Can you work these out from the drawing? Everything is in mm from the part's minimum corner. Round coordinates to 2 decimals unless told otherwise and drop trailing zeros. Order: outer loops, then holes, each group sorted by start corner. A loop starts at its lowest first (then second) coordinate and runs counter-clockwise, first axis right, second up. Notation, with made-up numbers: (74.25, 58.5) -> (115.25, 58.5) arc R28 cw to (115.25, 92.5) -> close; hole circle Ø7 at (-19.5, 80.5). An arc over 180 degrees is marked (long way). One line per item, written item: value.
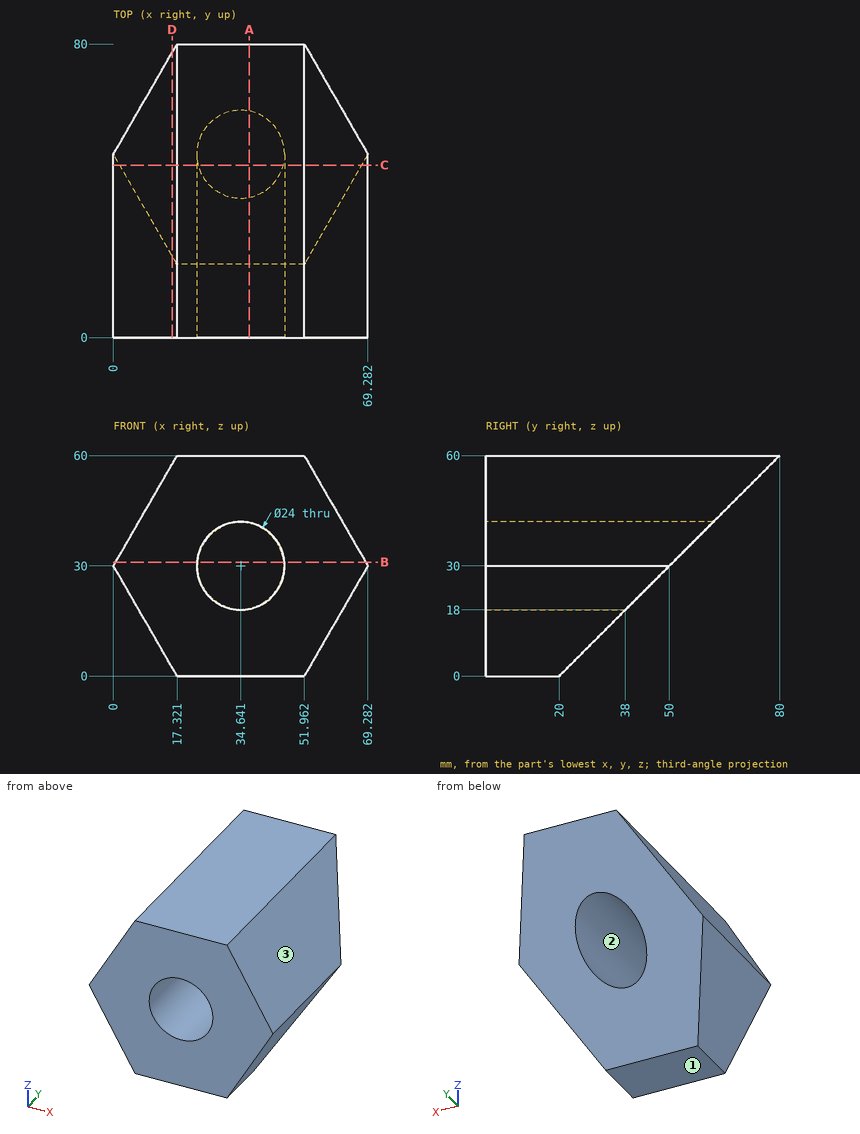
Q1. For P1, Ø4, axis at y = 19.5, z = 26, coming from the -X side (1 decimal); P2, Ø4, axis at x = 59, y = 58, coming from the -Z side; P3, Ø1, axis at x = 37.5, y = 36.5, coming from the -Z side; P4, Ø21.5, axis at x = 34.64, z = 30, coming from the -Y side, each with a flat end and sliding along its axis, tell me the tip position at first contact or that it passes through.
Answers:
P1: x = 1.2
P2: z = 36
P3: z = 16
P4: through
Q2. I want a section at C-C on y = 47. Write out the boundary of the cut face in (x, z), then the cut area to 3 significant figures.
Answers:
outline: (0, 30) -> (1.73, 27) -> (23.02, 27) arc R12 cw (long way) to (46.26, 27) -> (67.55, 27) -> (69.28, 30) -> (51.96, 60) -> (17.32, 60) -> close
area: 1,460 mm2
Q3. I need wall thicknesses on line 1 along X through (y, z) = (40.5, 30); line 2 along X through (y, z) = (29.5, 24.5) (1 decimal); line 3 along Z through (x, y) = (29, 28.5). Which ranges of each line are inside material? Lowest first, please.
Answers:
line 1: 0 to 22.64, 46.64 to 69.28
line 2: 3.2 to 24, 45.3 to 66.1
line 3: 8.5 to 19.41, 40.59 to 60
Q4. If we mould it in two halves opening along Z, with no side actions, what happens to the marked faces 1, 2 and 3? For each: pulls with the +Z half, pulls with the -Z half, needs draft (parallel to the pull), parting line crosses it, or undercut.
Answers:
face 1: pulls with the -Z half
face 2: undercut
face 3: pulls with the +Z half
Q5. I want a section at A-A on x = 37. Write out the boundary of the cut face in (y, z) (1 decimal), then the cut area to 3 significant figures.
Answers:
outline: (0, 0) -> (20, 0) -> (38.2, 18.2) -> (0, 18.2) -> close; (0, 41.8) -> (61.8, 41.8) -> (80, 60) -> (0, 60) -> close
area: 1,820 mm2
Q6. I want a section at B-B on z = 31. Write out the boundary of the cut face in (x, y) (1 decimal).
Answers:
outline: (0.6, 0) -> (22.7, 0) -> (22.7, 51) -> (0.6, 51) -> close; (46.6, 0) -> (68.7, 0) -> (68.7, 51) -> (46.6, 51) -> close
Q7. I want a section at D-D on x = 16. Write out the boundary of the cut face in (y, z), then the cut area to 3 significant figures.
Answers:
outline: (0, 2.29) -> (22.29, 2.29) -> (77.71, 57.71) -> (0, 57.71) -> close
area: 2,770 mm2
